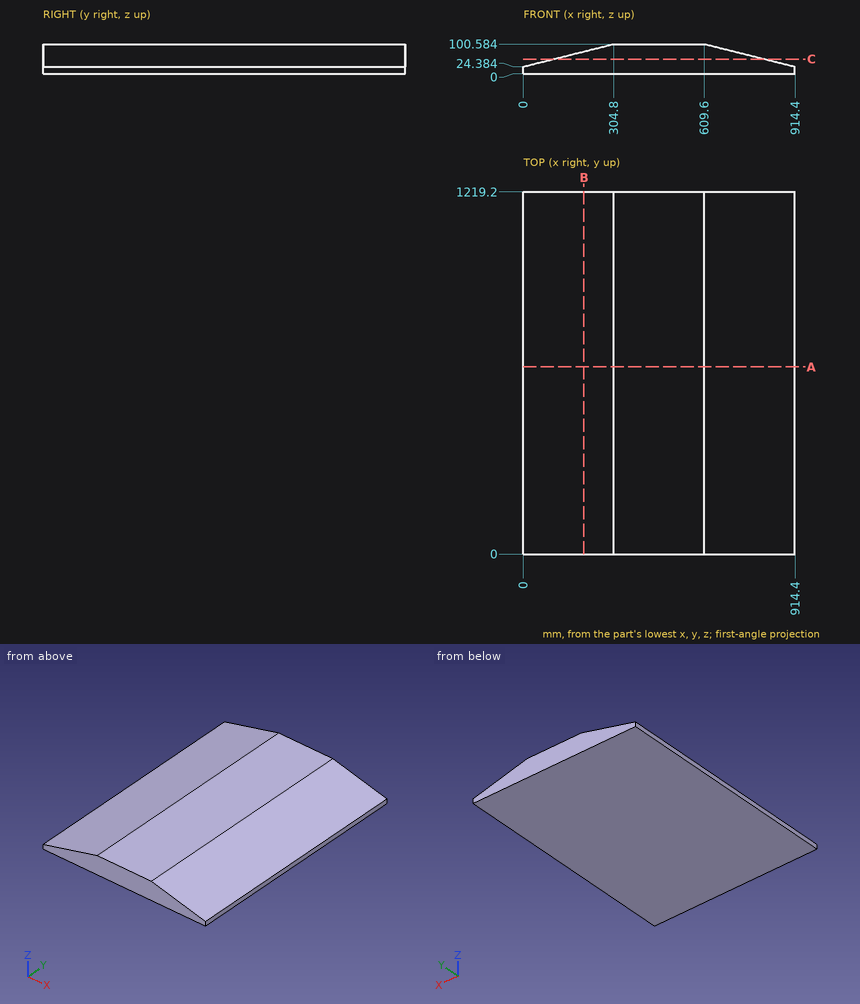
The drawing under review shows one solid part. Ordinate dimensions are in mm from its lowest x, y, z. Round coordinates to 2 decimals unless told otherwise and drop trailing zeros. Write each loop counter-clockwise with the first axis right and the second up, starting at its lowest first coordinate (ties: lowest second). Pieces come first, ordered by that corner, then holes. Notation, with made-up numbers: (-16.75, 46.25) - (1.25, 46.25) arc R18 cw to (1.25, 61.25) - close; hole circle Ø9 at (-12, -31). An arc over 180 degrees is marked (long way). Put each result on its own line as item: value.
Q1. We need section B-B (x = 204). Give the boundary of the cut face in (y, z), and give its area (3 significant figures).
Solved:
outline: (0, 0) - (1219.2, 0) - (1219.2, 75.38) - (0, 75.38) - close
area: 91,900 mm2
Q2. Wall thickness on probe 1 along Z at (x, y) = (654.5, 188); probe 2 along Z at (x, y) = (175, 310): over which ranges is each line inside the solid? List them lowest first.
Solved:
probe 1: z = 0 to 89.36
probe 2: z = 0 to 68.13
Q3. We need section A-A (y = 630.5). Give the boundary of the cut face in (x, z), and give its area (3 significant figures).
Solved:
outline: (0, 0) - (914.4, 0) - (914.4, 24.38) - (609.6, 100.58) - (304.8, 100.58) - (0, 24.38) - close
area: 68,700 mm2
Q4. We need section C-C (z = 50). Give the boundary of the cut face in (x, y).
Solved:
outline: (102.46, 0) - (811.94, 0) - (811.94, 1219.2) - (102.46, 1219.2) - close
